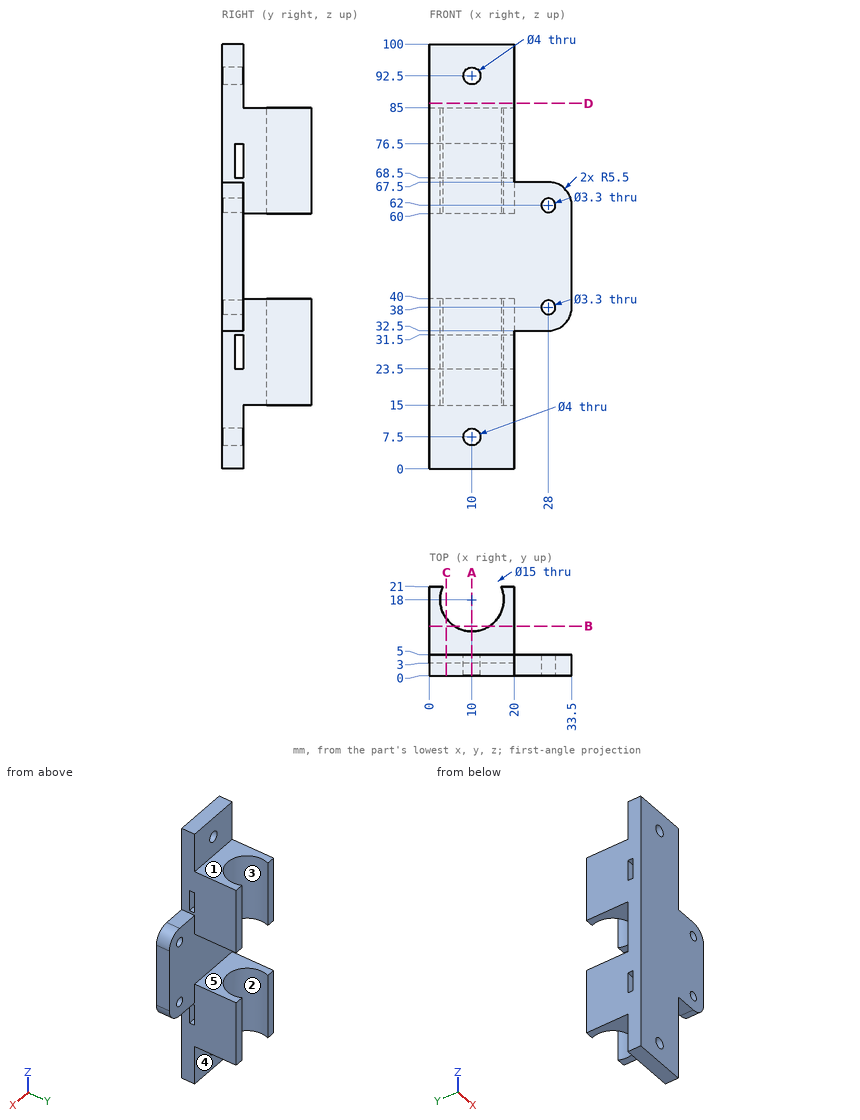
Drawing for the job (mm, zero at the part's lowest x, y, z). A direction names the side the tool comes from. Give positions to 0.01 mm unless a question says otherwise; leave off trailing zeros. Write each loop counter-clockwise with the first axis right and the second up, starting at its lowest first coordinate (ties: lowest second). Pieces come first, ordered by that corner, then holes. Notation, with made-up numbers: M 48,-13 L 63,-13 A14 ccw 63,2 Z; hole C 16.25,-28.75 d7. An arc over 180 degrees is marked long. Use CSV: the item, a comma, the result in double quotes.
Item 1: Slice it at A-A on x = 10. Write the cut outline in (y, z).
Taken from the geometry:
outline,"M 0,0 L 5,0 L 5,5.5 L 0,5.5 Z; M 0,9.5 L 5,9.5 L 5,15 L 10.5,15 L 10.5,40 L 5,40 L 5,60 L 10.5,60 L 10.5,85 L 5,85 L 5,90.5 L 0,90.5 Z; M 0,94.5 L 5,94.5 L 5,100 L 0,100 Z; hole M 3,23.5 L 5,23.5 L 5,31.5 L 3,31.5 Z; hole M 3,68.5 L 5,68.5 L 5,76.5 L 3,76.5 Z"
Item 2: Slice it at C-C on x = 4. Write the cut outline in (y, z).
Taken from the geometry:
outline,"M 0,0 L 5,0 L 5,15 L 13.5,15 L 13.5,40 L 5,40 L 5,60 L 13.5,60 L 13.5,85 L 5,85 L 5,100 L 0,100 Z; hole M 3,23.5 L 5,23.5 L 5,31.5 L 3,31.5 Z; hole M 3,68.5 L 5,68.5 L 5,76.5 L 3,76.5 Z"
Item 3: Which spindle directions (+Z, -Z, +X, -X, +Y, -Y) get a long thin tool onto all of the face, cutting with end or side? Do the marked faces 1 and 2. Say none if no direction does.
Taken from the geometry:
face 1,"+Z, +X, -X, +Y"
face 2,"+Z, -Z"
Item 4: Pin check, flat tips, straight feed: P1, Ø3, axis at y = 15, z = 33, coming from the +X side; P2, Ø5, axis at x = 10, z = 92.5, coming from the +Y side; P3, Ø1, axis at x = 10, y = 8, coming from the +Z side. Stop position of each tip, or through.
Taken from the geometry:
P1,"stops at x = 20"
P2,"stops at y = 5"
P3,"stops at z = 85"
Item 5: Drill centre lines: probe 1 along Z at (x, y) = (2, 11.5); probe 2 along X at (y, z) = (1.9, 62); probe 3 along X at (y, z) = (18, 34). Where is each one in solid material? Low to high.
Taken from the geometry:
probe 1,"z = 15 to 40, 60 to 85"
probe 2,"x = 0 to 26.35, 29.65 to 33.5"
probe 3,"x = 0 to 2.5, 17.5 to 20"
Item 6: Slice it at D-D on z = 86. Write the cut outline in (x, y), plus the area to 3 significant figures.
Taken from the geometry:
outline,"M 0,0 L 20,0 L 20,5 L 0,5 Z"
area,"100 mm²"
Item 7: Pull direction Y, two halves, no side cores. Call the marked faces 3, 4 and 5: +Y half, -Y half, draft (parallel to the pull), parting line (faces both ways), or undercut.
Taken from the geometry:
face 3,"undercut"
face 4,"+Y half"
face 5,"draft"
Item 8: Slice it at B-B on y = 11.75. Write the cut outline in (x, z).
Taken from the geometry:
outline,"M 0,15 L 5.85,15 L 5.85,40 L 0,40 Z; M 0,60 L 5.85,60 L 5.85,85 L 0,85 Z; M 14.15,15 L 20,15 L 20,40 L 14.15,40 Z; M 14.15,60 L 20,60 L 20,85 L 14.15,85 Z"
